Autodesk Inventor part; units mm, degrees
ref_plane "YZ Plane" through (0, 0, 0) normal (1, 0, 0) x (0, 1, 0)
ref_plane "XZ Plane" through (0, 0, 0) normal (0, 1, 0) x (-1, 0, 0)
ref_plane "XY Plane" through (0, 0, 0) normal (0, 0, 1) x (1, 0, 0)
sketch "Sketch1" plane through (0, 0, 0) normal (0, 1, 0) x (-1, 0, 0)
  circle A0 centre (0, 0) radius 5.85
  circle A1 centre (0, 0) radius 15
  dimension "d0" = 11.7
  dimension "d1" = 30
extrude "Extrusion1" add sketch "Sketch1" along normal blind 4.2
sketch "Sketch2" plane through (0, 4.2, 0) normal (0, 1, 0) x (1, 0, 0)
  circle A0 centre (0, 0) radius 15
extrude "Extrusion2" add sketch "Sketch2" along normal blind 3
shell "Shell1" thickness 1.5 removed faces 1 at (-11.748, 0, -1.6632)
sketch "Sketch3" plane through (0, 0, 0) normal (1, 0, 0) x (0, 1, 0)
  line L0 (5.7, -13.5) -> (5.7, 13.5)
  line L1 (5.7, 7.35) -> (0, 7.35)
  arc A0 (5.7, 13.5) -> (5.7, 7.35) centre (8.2582, 10.425) ccw
  line L2 (-1.6516, 0) -> (9.9098, 0)
  point P0 (0, 0)
  dimension "d7" = 4
revolve "Revolution1" add sketch "Sketch3" angle 360 about axis through (0, -10, 0) along (0, 1, 0)
fillet "Fillet1" radius 1.5 2 edges at (5.1969, 5.7, -5.1976) (-5.1969, 5.7, 5.1976)
properties part number "Button_adapter"
Geometry check sheet. Reference: the model listing, model coordinates, mm. A direction names the side the tool comes from. Give positions to 0.01 mm unless a question says otherwise; leave off trailing zeros. Loops run counter-clockwise (first coordinate to the right, second up) from the corner with the lowest first, then second, coordinate; pieces in that order, holes last. Notation, with made-up numbers: M 44.25,56.5 L 65.25,56.5 A19 cw 65.25,88.5 Z; hole C 14,27.25 d1. An arc over 180 degrees is marked long. Answer as CSV lines item,"result".
Item 1: Access from +Z, -Z, +X, -X, +Y, -Y to the whole of each face (thin tool, end or side, straight path). Record for faces 1 (the flat face through (0, 7.2, 0)), 2 (the flat face through (0, 4.2, 0)).
Values:
face 1,"+Z, -Z, +X, -X, +Y"
face 2,"-Y"
Item 2: Release check for a two-part mould opening along X. For faces 3 (the cylindrical face through (1.593, 1.474, 7.175)), 4 (the cylindrical face through (0.989, 4.35, 14.967)), 5 (the flat face through (1, 0, -6)) record: pulls with the +X half, pulls with the -X half, needs draft (parallel to the pull), parting line crosses it, or undercut.
Values:
face 3,"undercut"
face 4,"parting line crosses it"
face 5,"needs draft"
Item 3: Cross-section at A-A on y = 1.5. Record the cut outline in (x, z), and give its area (3 significant figures).
Values:
outline,"C 0,0 d30; C 0,0 d14.7; hole C 0,0 d27; hole C 0,0 d11.7"
area,"197 mm²"
Item 4: Material ranges on line 1 (Z direction, x = 0, y = 2.75); line 2 (Z direction, x = 4.5, y = 2.25); line 3 (Z direction, x = -11.25, y = 5.5), recorded low to high.
Values:
line 1,"z = -15 to -13.5, -7.35 to -5.85, 5.85 to 7.35, 13.5 to 15"
line 2,"z = -14.31 to -12.73, -5.81 to -3.74, 3.74 to 5.81, 12.73 to 14.31"
line 3,"z = -9.92 to -7.46, -7.14 to 7.14, 7.46 to 9.92"
Item 5: Depth check by flat-ended pin: P1, Ø1.5, axis at x = -2, y = 4, coming from the +Z side; P2, Ø6, axis at x = 1.5, z = 1.5, coming from the -Y side; P3, Ø2, axis at y = 4.5, z = 6, coming from the -X side. Enter the tip coordinate at first touch or a pass-through.
Values:
P1,"stops at z = 14.95"
P2,"stops at y = 4.2"
P3,"stops at x = -14.14"
Item 6: Cross-section at B-B on y = 5.25. Record the cut outline in (x, z), and give its area (3 significant figures).
Values:
outline,"C 0,0 d30; C 0,0 d26.12; hole C 0,0 d27"
area,"670 mm²"
